from build123d import *

# Parameters (mm, degrees)
CHAMFER2_SIZE         = 1
CHAMFER2_SIZE2        = 1.732050808
CHAMFER2_PART_2_SIZE  = 1
CHAMFER2_PART_2_SIZE2 = 1.732050808
FILLET1_R             = 1


with BuildPart() as part:
    # Sketch1 → Revolve1 (revolve)
    with BuildSketch(Plane.XY):
        Polygon((84.5, 60), (100, 60), (100, 0), (95, 0), (95, 5), (89.9, 5), (89.9, 0), (84.99, 0), (84.99, 19.369395797), (76.75, 30), (76.75, 35), (84.5, 35), align=None)
    revolve(axis=Axis((0, 0, 0), (0, 1, 0)))

    # Chamfer2
    chamfer2_edges = [part.edges().sort_by_distance(p)[0] for p in [
        (-84.5, 60, 0),
    ]]
    chamfer2_side = [part.faces().sort_by_distance(p)[0] for p in [
        (-84.5, 47.5, 0),
    ]]
    chamfer(chamfer2_edges, length=CHAMFER2_SIZE, length2=CHAMFER2_SIZE2, reference=chamfer2_side[0])

    # Chamfer2 part 2
    chamfer2_part_2_edges = [part.edges().sort_by_distance(p)[0] for p in [
        (-76.75, 35, 0),
    ]]
    chamfer2_part_2_side = [part.faces().sort_by_distance(p)[0] for p in [
        (-76.75, 32.5, 0),
    ]]
    chamfer(chamfer2_part_2_edges, length=CHAMFER2_PART_2_SIZE, length2=CHAMFER2_PART_2_SIZE2, reference=chamfer2_part_2_side[0])

    # Fillet1
    fillet1_edges = [part.edges().sort_by_distance(p)[0] for p in [
        (-95, 0, 0),
        (-89.9, 0, 0),
    ]]
    fillet(fillet1_edges, radius=FILLET1_R)


solid = part.part
The model under review builds one solid part; all positions refer to its coordinate system, in mm. A direction names the side the tool comes from. Round coordinates to 2 decimals unless told otherwise and drop trailing zeros. Write each loop counter-clockwise with the first axis right and the second up, starting at its lowest first coordinate (ties: lowest second). Pieces come first, ordered by that corner, then holes. Notation, with made-up numbers: M -37.75,-5 L -31.75,-5 A26 cw -31.75,11 Z; hole C 73.5,-21 d2. An arc over 180 degrees is marked long. Use a Markdown table: item, result. Add a question column.
Q1. Machinability: for faces 4 (the face through (-16.638, 32.028, 74.925)), 5 (the face through (-62.28, 47.17, -57.11)), 6 (the face through (-20.59, 3.03, 92.74)), which of the approach directions +Z, -Z, +X, -X, +Y, -Y give a long, thin tool a straight path to every point of the face, cutting with its end or side? Answer none if there is none.
Q2. We need section C-C, the plane y = 8.5. State the section outline as (x, z) points, plus the area to 3 significant figures.
Q3. Insertion check: pin 1 (10 mm diameter, centred on y = 41, z = 31, fed in from -X); pin 2 (4 mm diameter, centred on x = -58.5, y = 33.5, fed in from +Z); pin 3 (12 mm diameter, centred on y = 41.5, z = -51.5, fed in from +X). Each pin has a flat end and moves straight along its axis. Give the tip position at first contact, or say it passes through.
Q4. The part is to be moulded in two halves that separate along Z. For faces 1 (the face through (72, 0, 46)), 2 (the face through (-25, 35, 75)), 3 (the face through (95.38, 29.58, -30.04)), say which applies: pulls with the +Z half, pulls with the -Z half, needs draft (parallel to the pull), parting line crosses it, or undercut.
Q5. To check wall thickness, follow line 1 (Z direction, x = 0, y = 2.8); line 2 (X direction, y = 32, z = 0); line 3 (Z direction, x = 0, y = 9). State the ranges of each line that lie inside material, in increasing order.
Findings below:
| question | item | result |
|---|---|---|
| 1 | face 4 | +Y, -Y |
| 1 | face 5 | +Y |
| 1 | face 6 | -Y |
| 2 | outline | C 0,0 d200; hole C 0,0 d169.98 |
| 2 | area | 8,720 mm² |
| 3 | pin 1 | stops at x = -96.56 |
| 3 | pin 2 | stops at z = 82.51 |
| 3 | pin 3 | stops at x = 89.05 |
| 4 | face 1 | needs draft |
| 4 | face 2 | undercut |
| 4 | face 3 | parting line crosses it |
| 5 | line 1 | z = -100 to -95, -89.9 to -84.99, 84.99 to 89.9, 95 to 100 |
| 5 | line 2 | x = -100 to -76.75, 76.75 to 100 |
| 5 | line 3 | z = -100 to -84.99, 84.99 to 100 |
